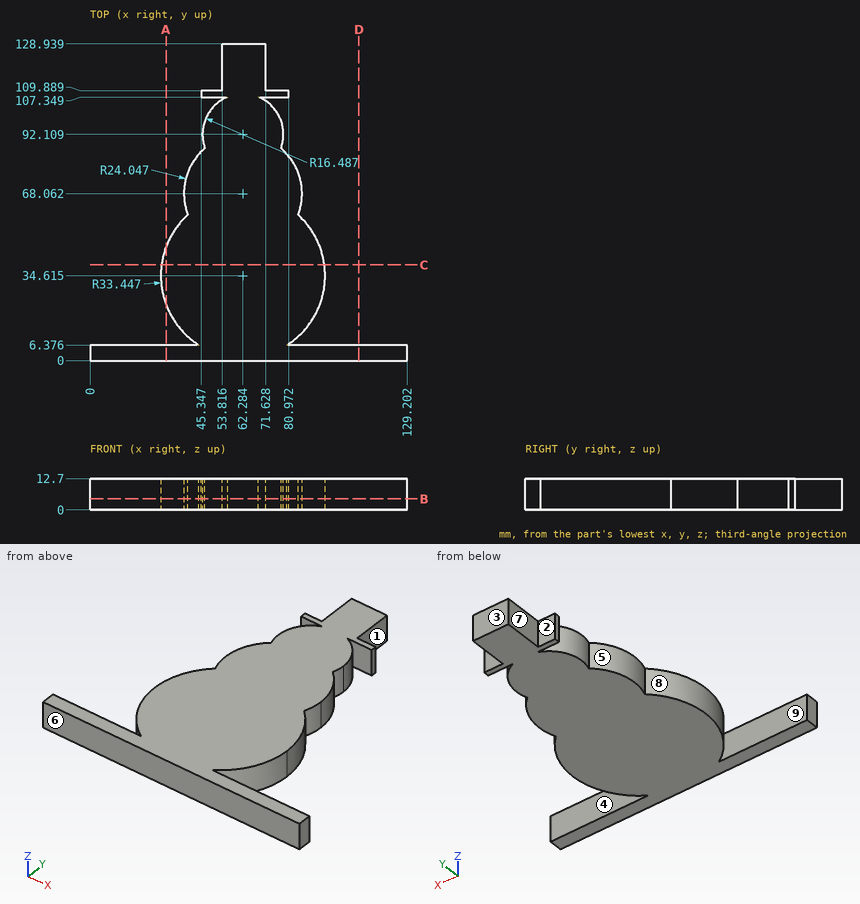
Verification items for this drawing (mm, ordinates from the low corner). A direction names the side the tool comes from. Coordinates: 2 decimals unless noted, no trailing zeros. Write each loop counter-clockwise with the first axis right and the second up, starting at its lowest first coordinate (ties: lowest second). Pieces come first, ordered by that corner, then holes. Notation, with made-up numbers: M 87,73.5 L 119,73.5 A22 ccw 119,106.5 Z; hole C 25.25,6 d4. An arc over 180 degrees is marked long. Answer as a JSON object with one key per item and string values. Group by question number.
(1) Release check for a two-part mould opening along Y. For the marked faces 6, 7, 8 and 9 record: +Y half, -Y half, draft (parallel to the pull), parting line (faces both ways), or undercut.
(2) Material ranges on line 1 (X direction, y = 113, z = 3) (1 decimal); line 2 (Y direction, x = 79, z = 7); line 3 (Y direction, x = 112, z = 10), recorded low to high.
(3) Cross-section at A-A, the plane x = 31. Record the cut outline in (y, z).
(4) Cross-section at C-C, the plane y = 39. Record the cut outline in (x, z) (1 decimal), and give its area (3 significant figures).
(5) Gauge pin test, flat ends, axial feed: pin 1 (1.5 mm diameter, centred on y = 113, z = 2.5, fed in from -X); pin 2 (4 mm diameter, centred on x = 19, z = 3, fed in from +Y); pin 3 (7 mm diameter, centred on x = 48.5, z = 8, fed in from +Y). Record the tip position at first contact, or that the pin passes through.
(6) Tool access check on the marked faces 1, 2, 3, 4 and 5. Record the directions out of +Z, -Z, +X, -X, +Y, -Y that give a thin tool (end or side, any length) a straight path to the whole face; none if there is none.
(7) Cross-section at D-D, the plane x = 109.5. Record the cut outline in (y, z).
(8) Cross-section at B-B, the plane z = 4.5. Record the cut outline in (x, y) (1 decimal), and give its area (3 significant figures).
Reply:
{
 "1": {"face 6": "-Y half", "face 7": "draft", "face 8": "undercut", "face 9": "undercut"},
 "2": {"line 1": "53.8 to 71.6", "line 2": "0 to 85.35, 107.35 to 109.89", "line 3": "0 to 6.38"},
 "3": {"outline": "M 0,0 L 6.38,0 L 6.38,12.7 L 0,12.7 Z; M 22.78,0 L 46.45,0 L 46.45,12.7 L 22.78,12.7 Z"},
 "4": {"outline": "M 29.1,0 L 95.4,0 L 95.4,12.7 L 29.1,12.7 Z", "area": "842 mm²"},
 "5": {"pin 1": "x = 53.82", "pin 2": "y = 6.38", "pin 3": "y = 109.89"},
 "6": {"face 1": "+Z, -Z, +X, +Y", "face 2": "+Z, -Z, -X, +Y", "face 3": "+Z, -Z, +X, -X, +Y", "face 4": "+Z, -Z, +X", "face 5": "+Z, -Z, -X"},
 "7": {"outline": "M 0,0 L 6.38,0 L 6.38,12.7 L 0,12.7 Z"},
 "8": {"outline": "M 0,0 L 129.2,0 L 129.2,6.4 L 80.2,6.4 A33.4 ccw 84.7,59.4 A24 ccw 77.8,86.5 A16.5 ccw 68.6,107.3 L 81,107.3 L 81,109.9 L 71.6,109.9 L 71.6,128.9 L 53.8,128.9 L 53.8,109.9 L 45.3,109.9 L 45.3,107.3 L 56,107.3 A16.5 ccw 46.8,86.5 A24 ccw 39.8,59.4 A33.4 ccw 44.4,6.4 L 0,6.4 Z", "area": "6,170 mm²"}
}
